CAD build for the part. Positions are in the model's coordinates, mm. A direction names the side the tool comes from. Round coordinates to 2 decimals unless told otherwise and drop trailing zeros. Order: outer loops, then holes, each group sorted by start corner. A loop starts at its lowest first (then second) coordinate and runs counter-clockwise, first axis right, second up. Notation, with made-up numbers: M 4,56.25 L 14,56.25 A16 cw 14,80.25 Z; hole C 76.25,-27 d11. An arc over 180 degrees is marked long. Answer as a JSON object with one key per item and string values.
```python
from build123d import *

# Parameters (mm, degrees)
SKETCH1_R                   = 8
BOSS_EXTRUDE1_DEPTH         = 5
SKETCH2_R                   = 8
BOSS_EXTRUDE2_DEPTH         = 10
BOSS_EXTRUDE2_TAPER         = 12
CUT_EXTRUDE5_DEPTH          = 19.788294313
CIRPATTERN1_COUNT           = 3
M5_TAPPED_HOLE1_D           = 4.2
M5_TAPPED_HOLE1_CSINK_D     = 5.05
M5_TAPPED_HOLE1_CSINK_ANGLE = 100
SKETCH6_W                   = 1.053506638
SKETCH6_H                   = 3.031369011


with BuildPart() as part:
    # Sketch1 → Boss-Extrude1 (new body)
    with BuildSketch(Plane(origin=(0, 0, 0), x_dir=(0, 0, -1), z_dir=(1, 0, 0))):
        Circle(SKETCH1_R)
    extrude(amount=BOSS_EXTRUDE1_DEPTH)

    # Sketch2 → Boss-Extrude2 (add)
    with BuildSketch(Plane(origin=(5, 0, 0), x_dir=(0, 0, -1), z_dir=(1, 0, 0))):
        Circle(SKETCH2_R)
    extrude(amount=BOSS_EXTRUDE2_DEPTH, taper=BOSS_EXTRUDE2_TAPER)

    # Sketch3 → Cut-Extrude5 (cut, through all)
    with BuildSketch(Plane(origin=(15, 0, 0), x_dir=(0, 0, -1), z_dir=(1, 0, 0))):
        with BuildLine():
            Line((0, 5.874434383), (11.406864113, 7.885772292))
            ThreePointArc((11.406864113, 7.885772292), (0.570239316, 16.679095968), (-10.070915149, 7.650208444))
            Line((-10.070915149, 7.650208444), (0, 5.874434383))
        make_face()
    cut_extrude5 = extrude(amount=-CUT_EXTRUDE5_DEPTH, mode=Mode.SUBTRACT)

    # CirPattern1: Cut-Extrude5 ×3 about axis
    cirpattern1_axis = Axis((0, 0, 0), (1, 0, 0))
    for i in range(1, CIRPATTERN1_COUNT):
        add(cut_extrude5.rotate(cirpattern1_axis, i * 360 / CIRPATTERN1_COUNT), mode=Mode.SUBTRACT)

    # M5 Tapped Hole1 (through all)
    with Locations(Plane(origin=(15, 0, 0), x_dir=(0, 0, -1), z_dir=(1, 0, 0))):
        with Locations((0, 0)):
            CounterSinkHole(M5_TAPPED_HOLE1_D / 2, M5_TAPPED_HOLE1_CSINK_D / 2, counter_sink_angle=M5_TAPPED_HOLE1_CSINK_ANGLE)

    # Sketch6 → Cut-Revolve2 (revolve, cut)
    with BuildSketch(Plane.XY, mode=Mode.PRIVATE) as cut_revolve2_sk:
        with Locations((2.120528078, 7.390118889)):
            Rectangle(SKETCH6_W, SKETCH6_H)
    revolve(cut_revolve2_sk.sketch.rotate(Axis((0, 0, 0), (1, 0, 0)), 270), axis=Axis((0, 0, 0), (1, 0, 0)), mode=Mode.SUBTRACT)


solid = part.part
```
Item 1: Wall check: line 1 along Y through (x, z) = (3.25, 0); line 2 along Z through (x, y) = (12, 0); line 3 along Z through (x, y) = (8.25, 0). Give the ranges that are in metal, low to high. Write a range as [from, to].
Worked answers:
{"line 1": "y = [-8, -2.1], [2.1, 5.87]", "line 2": "z = [-6.51, -2.1], [2.1, 6.51]", "line 3": "z = [-7.31, -2.1], [2.1, 7.31]"}
Item 2: Saw through at C-C on x = 6.5. List the corners of the cut face in (y, z).
Worked answers:
{"outline": "M -6.73,-3.71 L -2.94,-5.09 L 0.15,-7.68 A7.68 ccw 6.57,-3.97 L 5.87,0 L 6.57,3.97 A7.68 ccw 0.15,7.68 L -2.94,5.09 L -6.73,3.71 A7.68 ccw Z; hole C 0,0 d4.2"}
Item 3: Two-plate mould, pull along X, no slides. Class faces 4 (the flat face through (2.647, -7, 0)), 5 (the flat face through (0, -2, -2)), 6 (the cylindrical face through (3.807, 4.044, 6.902)): released by +X, released by -X, zero draft, split by the parting line, or undercut.
Worked answers:
{"face 4": "undercut", "face 5": "released by -X", "face 6": "zero draft"}
Item 4: Saw through at B-B on y = 0. List the corners of the cut face in (x, z) (3 decimals), and give its area (3 significant figures).
Worked answers:
{"outline": "M 0,-7.552 L 1.594,-7.552 L 1.594,-5.874 L 2.647,-5.874 L 2.647,-7.552 L 7.108,-7.552 L 15,-5.874 L 15,-2.525 L 14.643,-2.1 L 0,-2.1 Z; M 0,2.1 L 14.643,2.1 L 15,2.525 L 15,5.874 L 7.108,7.552 L 2.647,7.552 L 2.647,5.874 L 1.594,5.874 L 1.594,7.552 L 0,7.552 Z", "area": "147 mm2"}
Item 5: Drop flat-ended pins along their axis: pin 1 Ø4 at (x, y) = (9.5, 0.5) entering from +Z; pin 2 Ø4 at (x, y) = (6, 2.5) entering from -Z; pin 3 Ø6 at (x, z) = (6.5, 0) entering from +Y. Give the stop position or say it passes through.
Worked answers:
{"pin 1": "stops at z = 7.46", "pin 2": "stops at z = -7.96", "pin 3": "stops at y = 6.4"}
Item 6: Saw through at A-A on x = 11.5. List the corners of the cut face in (y, z), and give its area (3 significant figures).
Worked answers:
{"outline": "M -5,-4.34 L -2.94,-5.09 L -1.26,-6.5 A6.62 ccw 6.26,-2.16 L 5.87,0 L 6.26,2.16 A6.62 ccw -1.26,6.5 L -2.94,5.09 L -5,4.34 A6.62 ccw Z; hole C 0,0 d4.2", "area": "118 mm2"}
Item 7: 3-axis set-ups, long thin cutter, end or side, ignore diameter. For faces 1 (the cylindrical face through (2.128, 5.824, 0.765)), 2 (the flat face through (7.538, 6.184, 1.757)), 3 (the flat face through (0.808, -1.236, 6.515)): which of +Z, -Z, +X, -X, +Y, -Y reach the whole face in a straight line?
Worked answers:
{"face 1": "none", "face 2": "+X, -X, +Y", "face 3": "+Z, +X, -X, -Y"}
